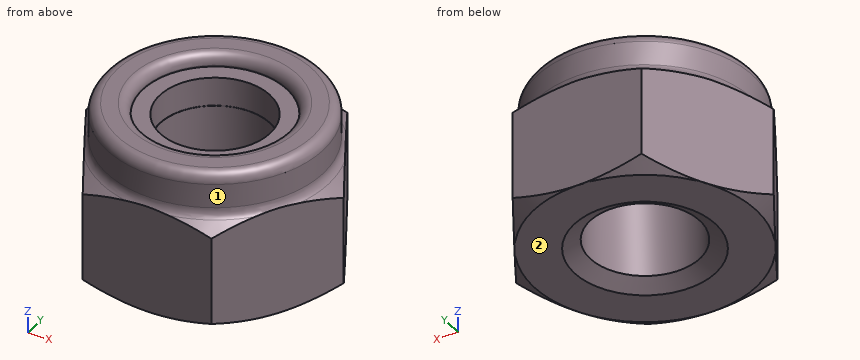
Solid Edge part; units mm, degrees
sketch "Sketch1" plane through (0, 0, 0) normal (0, 0, 1) x (1, 0, 0)
  circle A0 centre (0, 0) radius 4.188
  circle A1 centre (0, 0) radius 9.815
extrude "Protrusion1" add sketch "Sketch1" along normal blind 11.5
sketch "Sketch2" plane through (0, 0, 0) normal (0, 0, 1) x (1, 0, 0)
  line L0 (9.815, 0) -> (4.9075, 8.5)
  arc A0 (4.9075, 8.5) -> (9.815, 0) centre (0, 0) cw
extrude "ExtrudedCutout_1" cut sketch "Sketch2" along normal blind 11.5
pattern_circular "Pattern1" count 6 over 360 about axis through (0, 0, 0) along (0, 0, -1) of "ExtrudedCutout_1"
cosmetic_thread "Thread_1" thread depth 8.4
sketch "Sketch3" plane through (0, 0, 0) normal (0, -1, 0) x (1, 0, 0)
  line L0 (9.8153, 0.7666) -> (9.8153, 0)
  line L1 (9.8153, 0) -> (8.4875, 0)
  line L2 (8.4875, 0) -> (9.8153, 0.7666)
  line L3 (8.25, 11.5) -> (8.25, 8.8619)
  arc A0 (8.25, 8.8619) -> (8.65, 8.1691) centre (9.05, 8.8619) ccw
  line L4 (8.65, 8.1691) -> (9.8153, 7.4963)
  line L5 (9.8153, 7.4963) -> (9.8153, 11.5)
  line L6 (9.8153, 11.5) -> (8.25, 11.5)
  dimension "D1" = 8.25
revolve "RevolvedCutout_1" cut sketch "Sketch3" angle 360 about axis through (0, 0, 11.9) along (0, 0, -1)
sketch "Sketch4" plane through (0, 0, 0) normal (0, -1, 0) x (1, 0, 0)
  line L0 (4.188, 11.5) -> (4.188, 8.4)
  line L1 (5.5, 11.5) -> (4.188, 11.5)
  line L2 (5.5, 10.6) -> (5.5, 11.5)
  line L3 (4.213, 10.6) -> (5.5, 10.6)
  line L4 (4.213, 10.6) -> (4.213, 8.4)
  line L5 (4.213, 8.4) -> (4.188, 8.4)
  dimension "D1" = 5.5
  dimension "D2" = 4.188
  dimension "D3" = 4.213
revolve "RevolvedCutout_2" cut sketch "Sketch4" angle 360 about axis through (0, 0, 8.4) along (0, 0, -1)
fillet "Round_1" radius 0.8 2 edges at (-8.25, 0, 11.5) (-5.5, 0, 11.5)
chamfer "Chamfer_1" distance 1.212 angle 30 1 edges at (-4.188, 0, 0) measured on face at (-5.8281, -5.4886, 0)
properties material "Steel"
Geometry check sheet. Reference: the model listing, model coordinates, mm. Face numbers are marked on the shaded views. A direction names the side the tool comes from. Round coordinates to 2 decimals unless told otherwise and drop trailing zeros.
Item 1: Gauge pin test, flat ends, axial feed: pin 1 (4 mm diameter, centred on x = 7.5, z = 6.5, fed in from +Y); pin 2 (6.5 mm diameter, centred on x = 2, y = 1.5, fed in from +Z); pin 3 (3 mm diameter, centred on y = -3.5, z = 9, fed in from +X); pin 4 (7.5 mm diameter, centred on x = 0, y = 0, fed in from +Z). Record the tip position at first contact, or that the pin passes through.
Item 2: Thickness scan on line 1 (Y direction, x = 0, z = 9); line 2 (Y direction, x = 0, z = 10.65). Record the ranges inside material, lowest first.
Item 3: Access from +Z, -Z, +X, -X, +Y, -Y to the whole of each face (thin tool, end or side, straight path). Record for the marked faces 1 and 2.
Answer sheet:
1. pin 1: stops at y = 7.47
1. pin 2: stops at z = 11.28
1. pin 3: stops at x = 8.48
1. pin 4: passes through
2. line 1: y = -8.25 to -4.21, 4.21 to 8.25
2. line 2: y = -8.25 to -5.5, 5.5 to 8.25
3. face 1: +Z
3. face 2: -Z, +X, -X, +Y, -Y
